The listing builds one solid part. Answer for the finished solid, in the listing's coordinates (mm). Coordinates: 2 decimals unless noted, no trailing zeros. Write each loop counter-clockwise with the first axis right and the second up, starting at its lowest first coordinate (ties: lowest second). Pieces come first, ordered by that corner, then holes. Notation, with made-up numbers: M 43.5,18 L 73.5,18 A30 ccw 73.5,42 Z; hole C 25.5,15.5 d5. An arc over 180 degrees is marked long. Answer as CSV lines item,"result". Start each with the question number.
```python
from build123d import *

# Parameters (mm, degrees)
F0_R     = 3.683
F1_DEPTH = 3.175


with BuildPart() as f1:
    # F0 (on Top) → F1 (new body)
    with BuildSketch(Plane.XY):
        with BuildLine():
            ThreePointArc((0, 6.35), (1.859872, 1.859872), (6.35, 0))
            Line((6.35, 0), (44.45, 0))
            ThreePointArc((44.45, 0), (48.940128, 1.859872), (50.8, 6.35))
            Line((50.8, 6.35), (50.8, 171.45))
            ThreePointArc((50.8, 171.45), (48.940128, 175.940128), (44.45, 177.8))
            Line((44.45, 177.8), (6.35, 177.8))
            ThreePointArc((6.35, 177.8), (1.859872, 175.940128), (0, 171.45))
            Line((0, 171.45), (0, 6.35))
        make_face()
        with Locations((38.1, 12.7)):
            Circle(F0_R, mode=Mode.SUBTRACT)
        with Locations((38.1, 25.4)):
            Circle(F0_R, mode=Mode.SUBTRACT)
        with Locations((38.1, 38.1)):
            Circle(F0_R, mode=Mode.SUBTRACT)
        with Locations((38.1, 50.8)):
            Circle(F0_R, mode=Mode.SUBTRACT)
        with Locations((38.1, 63.5)):
            Circle(F0_R, mode=Mode.SUBTRACT)
        with Locations((38.1, 76.2)):
            Circle(F0_R, mode=Mode.SUBTRACT)
        with Locations((38.1, 88.9)):
            Circle(F0_R, mode=Mode.SUBTRACT)
        with Locations((38.1, 101.6)):
            Circle(F0_R, mode=Mode.SUBTRACT)
        with Locations((38.1, 114.3)):
            Circle(F0_R, mode=Mode.SUBTRACT)
        with Locations((38.1, 127)):
            Circle(F0_R, mode=Mode.SUBTRACT)
        with Locations((38.1, 139.7)):
            Circle(F0_R, mode=Mode.SUBTRACT)
        with Locations((38.1, 152.4)):
            Circle(F0_R, mode=Mode.SUBTRACT)
        with Locations((38.1, 165.1)):
            Circle(F0_R, mode=Mode.SUBTRACT)
    extrude(amount=F1_DEPTH)


solid = f1.part
```
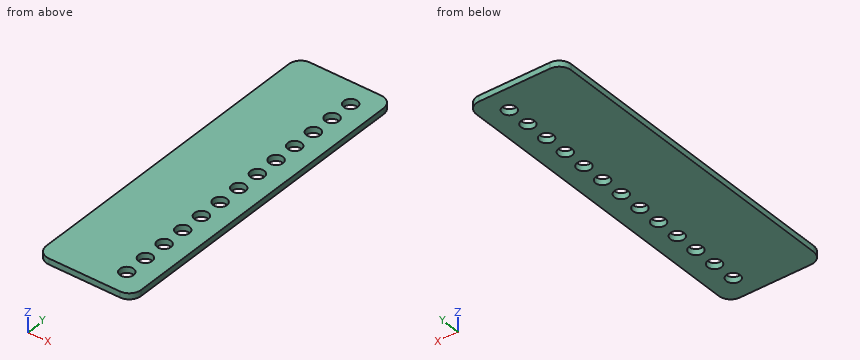
1) Each of these flat-tipped pins is pushed along its axis until it touches: P1, Ø4, axis at x = 11, y = 156.5, coming from the -Z side; P2, Ø1, axis at x = 45.5, z = 1, coming from the -Y side. Where does it stop, or does it pass through?
2) The part is cut by section A-A (z = 1.4). Count the separate pieces of the cut face and the enclosed holes in it, then the cut area to 3 significant figures.
3) Find the intervals of material crossed by line 1 (X direction, y = 165.1, z = 0.9); line 2 (X direction, y = 128, z = 1.95); line 3 (Y direction, x = 2.5, z = 0.4), in increasing order. Write a range as from..to.
4) The part is cut by section D-D (y = 125.5). Determine the outline of the cut face in (x, z) (3 decimals), then the cut area to 3 significant figures.
5) The part is cut by section B-B (y = 165.1). Determine the outline of the cut face in (x, z) (3 decimals).
Completed:
1,P1,"z = 0"
1,P2,"y = 0.02"
2,separate pieces,"1"
2,enclosed holes,"13"
2,area,"8,440 mm²"
3,line 1,"0..34.42, 41.78..50.8"
3,line 2,"0..34.56, 41.64..50.8"
3,line 3,"1.3..176.5"
4,outline,"M 0,0 L 34.736,0 L 34.736,3.175 L 0,3.175 Z; M 41.464,0 L 50.8,0 L 50.8,3.175 L 41.464,3.175 Z"
4,area,"140 mm²"
5,outline,"M 0,0 L 34.417,0 L 34.417,3.175 L 0,3.175 Z; M 41.783,0 L 50.8,0 L 50.8,3.175 L 41.783,3.175 Z"
